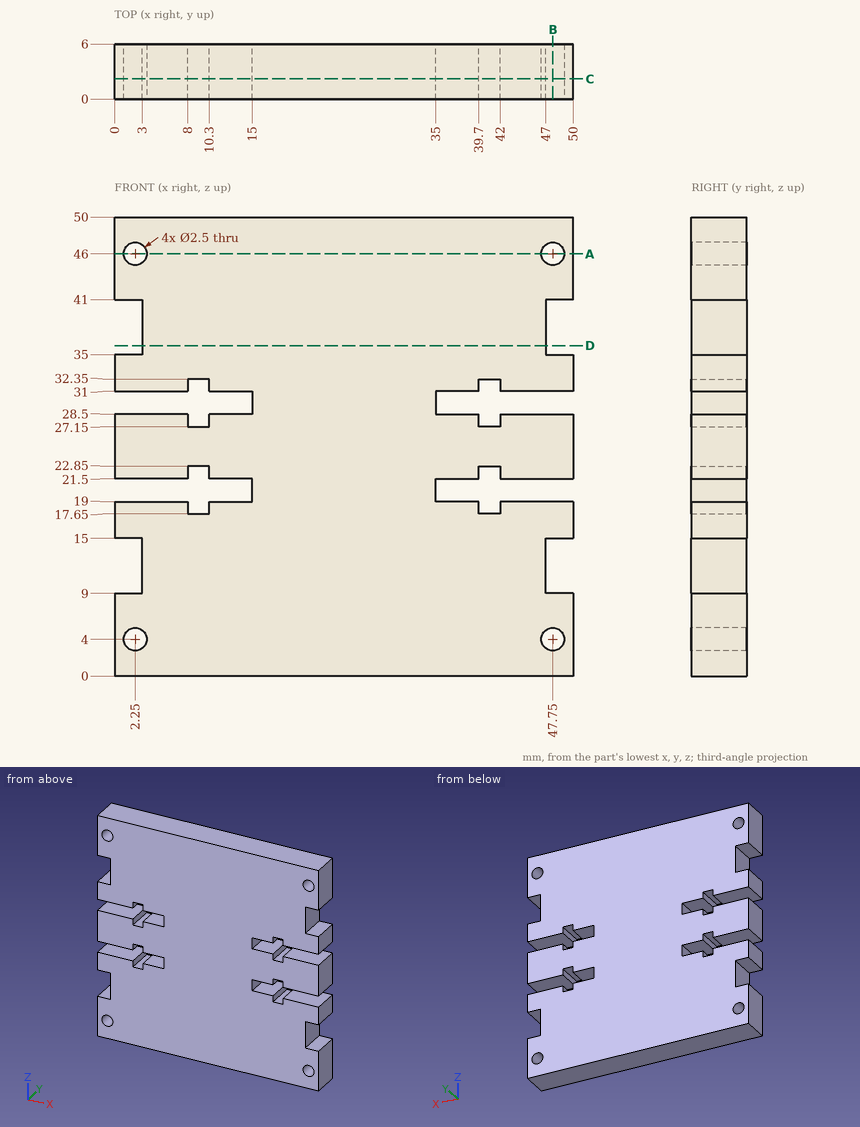
Study the drawing (mm; zero at the part's minimum x, y, z) and answer. Coordinates: 2 decimals unless noted, no trailing zeros. Loops run counter-clockwise (first coordinate to the right, second up) from the corner with the lowest first, then second, coordinate; pieces in that order, holes last. Notation, with made-up numbers: (82, 47.25) -> (131, 47.25) arc R22 cw to (131, 58.25) -> close; hole circle Ø1 at (55.5, 6). An arc over 180 degrees is marked (long way). Write item = value, one per line. Start each with the question number.
1) Given P1, Ø0.8, axis at y = 3.5, z = 30, coming from the -X side, flat-ended and moving along its own axis, determine where the tip first touches the part or whether it passes through.
2) The part is cut by section C-C, the plane y = 2.2. State how many separate pieces and enclosed holes the cut face has, plus the area to 3 significant figures.
3) The part is cut by section B-B, the plane x = 47.75. Determine the outline of the cut face in (y, z), plus the area to 3 significant figures.
4) The part is cut by section D-D, the plane z = 36. Determine the outline of the cut face in (x, y).
5) The part is cut by section A-A, the plane z = 46. Determine the outline of the cut face in (x, y), plus the area to 3 significant figures.
6) Find the intervals of material crossed by L1, parallel to X at y = 0.8, z = 32; L2, parallel to Z at x = 40, y = 1.1; L3, parallel to X at y = 1.6, z = 14, in increasing order. Write a range as from..to.
Result:
q1.P1 = 15
q2.separate_pieces = 1
q2.enclosed_holes = 4
q2.area = 2,230 mm²
q3.outline = (0, 0) -> (6, 0) -> (6, 2.75) -> (0, 2.75) -> close; (0, 5.25) -> (6, 5.25) -> (6, 9) -> (0, 9) -> close; (0, 15) -> (6, 15) -> (6, 19) -> (0, 19) -> close; (0, 21.5) -> (6, 21.5) -> (6, 28.5) -> (0, 28.5) -> close; (0, 31) -> (6, 31) -> (6, 35) -> (0, 35) -> close; (0, 41) -> (6, 41) -> (6, 44.75) -> (0, 44.75) -> close; (0, 47.25) -> (6, 47.25) -> (6, 50) -> (0, 50) -> close
q3.area = 168 mm²
q4.outline = (3, 0) -> (47, 0) -> (47, 6) -> (3, 6) -> close
q5.outline = (0, 0) -> (1, 0) -> (1, 6) -> (0, 6) -> close; (3.5, 0) -> (46.5, 0) -> (46.5, 6) -> (3.5, 6) -> close; (49, 0) -> (50, 0) -> (50, 6) -> (49, 6) -> close
q5.area = 270 mm²
q6.L1 = 0..8, 10.3..39.7, 42..50
q6.L2 = 0..17.65, 22.85..27.15, 32.35..50
q6.L3 = 3..47
